Read the model definition and answer for the solid it produces. Units are mm, in the model's axes. A direction names the side the tool comes from. Coordinates: 2 decimals unless noted, no trailing zeros. Order: outer loops, then holes, each group sorted by start corner. A loop starts at its lowest first (then second) coordinate and runs counter-clockwise, first axis right, second up. Notation, with made-up numbers: (-25.5, 23) -> (33.5, 23) arc R13 ccw to (33.5, 40) -> close; hole circle Ø2 at (38, 13). An arc over 180 degrees is marked (long way). Answer as a JSON object with one key per item and string values. Group by question number.
1) Consider L1, parallel to X at y = 38.5, z = -31.5; L2, parallel to Z at x = 1.5, y = 16.5; L3, parallel to Z at x = 26, y = 13.5. Determine where each line is inside the solid, lowest interval first.
2) Section B-B on y = 15 is taken. Determine the outline of the cut face in (x, z).
3) Section D-D on y = 44 is taken. Determine the outline of the cut face in (x, z).
4) Section A-A on z = 0 is taken. Determine the outline of the cut face in (x, y).
5) A tool of negligible diameter and unlimited length cuts with its end or side. For faces 4 (the flat face through (-68, 27, -15)), 5 (the cylindrical face through (-29.791, -15.513, -29.605)), 6 (the flat face through (66.17, -38.9, -26.59)), 7 (the cylindrical face through (-79.832, -8.071, -61.472)), from which of +Z, -Z, +X, -X, +Y, -Y can it reach the whole face along a straight path? Write none if from no direction.
6) Section C-C on x = -51 is taken. Determine the outline of the cut face in (y, z), and give its area (3 significant figures).
7) Given pin 1 (2 mm diameter, centred on x = -19.5, z = 19, fed in from +Y); pin 2 (1.5 mm diameter, centred on y = -4.5, z = -22.5, fed in from +X); pin 3 (2 mm diameter, centred on x = -27, y = -6.5, fed in from +Z), each flat-ended and moving along its own axis, determine where each tip first touches the part or whether it passes through.
8) Determine the mould class of faces 1 (the flat face through (-27, -20, -28)), 2 (the flat face through (-92, 1, -1)), 3 (the flat face through (78, -74, 1)) for opening direction X: released by +X, released by -X, zero draft, split by the parting line, or undercut.
from build123d import *

# Parameters (mm, degrees)
SKETCH2_W           = 42
SKETCH2_H           = 60
SKETCH3_R           = 33
BOSS_EXTRUDE1_DEPTH = 24
SKETCH6_W           = 62
SKETCH6_H           = 30


with BuildPart() as part:
    # Sketch1 → Revolve1 (revolve)
    with BuildSketch(Plane.XY):
        Polygon((-92, 0), (-92, 62), (-68, 62), (-68, 30), (0, 30), (0, 0), align=None)
    revolve(axis=Axis((0, 0, 0), (-1, 0, 0)))

    # Sketch2 → Revolve2 (revolve)
    with BuildSketch(Plane(origin=(0, 0, 0), x_dir=(0, 0, -1), z_dir=(1, 0, 0))):
        with Locations((21, 10)):
            Rectangle(SKETCH2_W, SKETCH2_H)
    revolve(axis=Axis((0, 40, 0), (0, -1, 0)))

    # Sweep1: sweep along a path in Sketch4
    with BuildLine(Plane.XY) as sweep1_path:
        Line((0, -20), (0, -37))
        ThreePointArc((0, -37), (11.129942315, -63.870057685), (38, -75))
        Line((38, -75), (78, -75))
    # Sketch3 → Sweep1 (sweep)
    with BuildSketch(Plane.XZ.offset(20)):
        Circle(SKETCH3_R)
    sweep(path=sweep1_path.line)

    # Sketch5 → Boss-Extrude1 (add)
    with BuildSketch(Plane(origin=(78, 0, 0), x_dir=(0, 0, -1), z_dir=(1, 0, 0))):
        with BuildLine():
            Line((-19.364916731, -20), (-33.616565645, -57.282028495))
            ThreePointArc((-33.616565645, -57.282028495), (-38, -75), (-33.616565645, -92.717971505))
            Line((-33.616565645, -92.717971505), (-19.364916731, -130))
            ThreePointArc((-19.364916731, -130), (0, -145), (19.364916731, -130))
            Line((19.364916731, -130), (33.616565645, -92.717971505))
            ThreePointArc((33.616565645, -92.717971505), (38, -75), (33.616565645, -57.282028495))
            Line((33.616565645, -57.282028495), (19.364916731, -20))
            ThreePointArc((19.364916731, -20), (0, -5), (-19.364916731, -20))
        make_face()
    extrude(amount=-BOSS_EXTRUDE1_DEPTH)

    # Sketch6 → Revolve3 (revolve)
    with BuildSketch(Plane(origin=(0, 0, 0), x_dir=(0, 0, -1), z_dir=(1, 0, 0))):
        with Locations((31, 15)):
            Rectangle(SKETCH6_W, SKETCH6_H)
    revolve(axis=Axis((0, 0, 0), (0, 0, -1)))


solid = part.part
Worked answers:
{
 "1": {"L1": "x = -92 to -68, -27.78 to 27.78", "L2": "z = -62 to 41.97", "L3": "z = -62 to 32.98"},
 "2": {"outline": "(-92, -60.16) -> (-68, -60.16) -> (-68, -25.98) -> (-33, -25.98) arc R42 ccw to (-25.98, -33) -> (-25.98, -62) -> (25.98, -62) -> (25.98, -33) arc R42 ccw (long way) to (-33, 25.98) -> (-68, 25.98) -> (-68, 60.16) -> (-92, 60.16) -> close"},
 "3": {"outline": "(-92, -43.68) -> (-68, -43.68) -> (-68, 43.68) -> (-92, 43.68) -> close"},
 "4": {"outline": "(-92, -62) -> (-68, -62) -> (-68, -30) -> (-33, -30) -> (-33, -37) arc R71 ccw to (38, -108) -> (54, -108) -> (54, -145) -> (78, -145) -> (78, -5) -> (54, -5) -> (54, -42) -> (38, -42) arc R5 cw to (33, -37) -> (33, -20) -> (42, -20) -> (42, 40) -> (-42, 40) -> (-42, 30) -> (-68, 30) -> (-68, 62) -> (-92, 62) -> close"},
 "5": {"face 4": "none", "face 5": "-Z, -Y", "face 6": "-Z, +X, +Y", "face 7": "-X"},
 "6": {"outline": "circle Ø60 at (0, 0)", "area": "2,830 mm²"},
 "7": {"pin 1": "stops at y = 40", "pin 2": "stops at x = 35.93", "pin 3": "stops at z = 32.98"},
 "8": {"face 1": "undercut", "face 2": "released by -X", "face 3": "released by +X"}
}
